Geometry check sheet. Reference: drawing and pictorial views, mm from the part's lowest x, y, z. A direction names the side the tool comes from. Coordinates: 2 decimals unless noted, no trailing zeros. Write each loop counter-clockwise with the first axis right and the second up, starting at its lowest first coordinate (ties: lowest second). Pieces come first, ordered by that corner, then holes. Notation, with made-up numbers: (16, 37) - (74, 37) arc R19 ccw to (74, 43) - close; hole circle Ø6 at (-14, -38). An arc over 180 degrees is marked (long way). Answer as CSV lines item,"result". Start each with the question number.
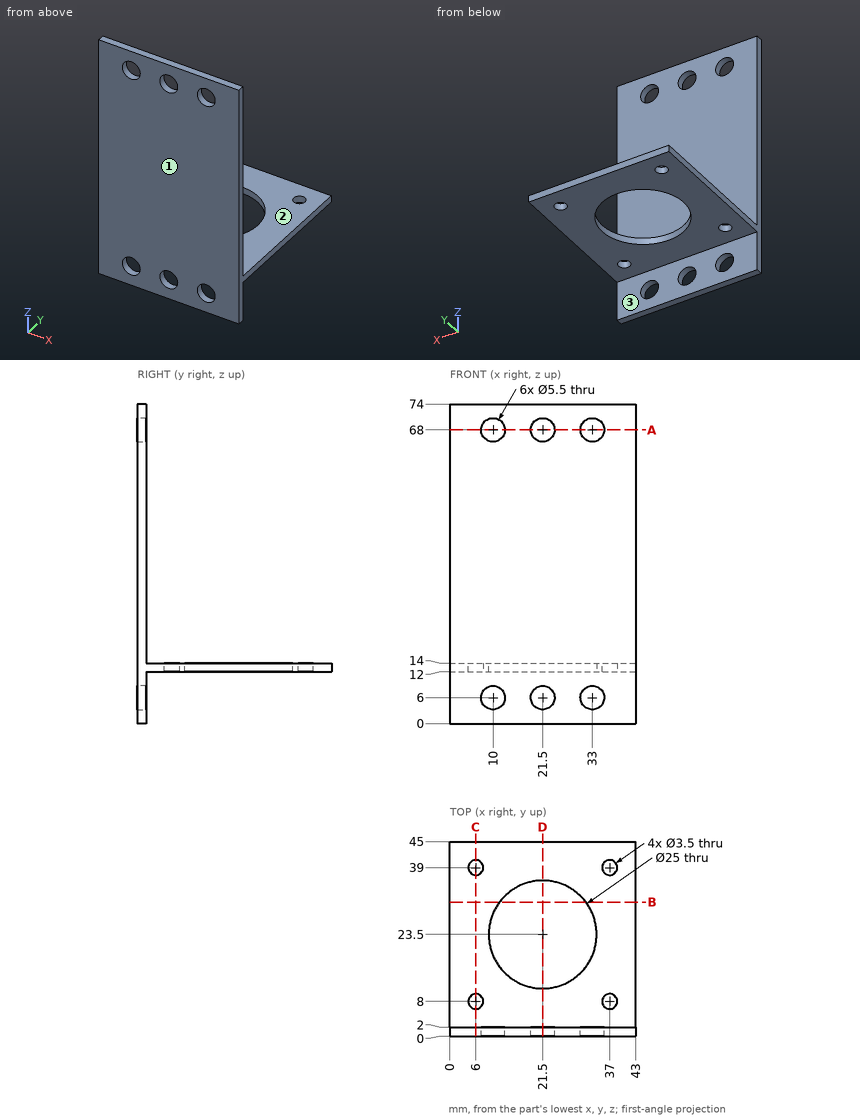
1. Cross-section at C-C (x = 6). Record the cut outline in (y, z).
2. Cross-section at A-A (z = 68). Record the cut outline in (x, y).
3. Cross-section at D-D (x = 21.5). Record the cut outline in (y, z).
4. Cross-section at B-B (y = 31). Record the cut outline in (x, z), and give its area (3 significant figures).
5. Depth check by flat-ended pin: P1, Ø10, axis at x = 13, z = 9.5, coming from the +Y side; P2, Ø13, axis at x = 19, y = 33, coming from the -Z side; P3, Ø21.5, axis at x = 14, y = 18.5, coming from the +Z side; P4, Ø7, axis at x = 33, z = 68, coming from the +Y side. Enter the tip coordinate at first touch or a pass-through.
6. Scan lines: line 1 along X through (y, z) = (0.6, 6); line 2 along Y through (x, z) = (37, 13.3); line 3 along Z through (x, y) = (8, 19.5). Record each from-to range of solid material in increasing order. Write a range as from..to.
7. Access from +Z, -Z, +X, -X, +Y, -Y to the whole of each face (thin tool, end or side, straight path). Record for the marked faces 1, 2 and 3.
Completed:
1,outline,"(0, 0) - (2, 0) - (2, 12) - (6.25, 12) - (6.25, 14) - (2, 14) - (2, 74) - (0, 74) - close; (9.75, 12) - (37.25, 12) - (37.25, 14) - (9.75, 14) - close; (40.75, 12) - (45, 12) - (45, 14) - (40.75, 14) - close"
2,outline,"(0, 0) - (7.25, 0) - (7.25, 2) - (0, 2) - close; (12.75, 0) - (18.75, 0) - (18.75, 2) - (12.75, 2) - close; (24.25, 0) - (30.25, 0) - (30.25, 2) - (24.25, 2) - close; (35.75, 0) - (43, 0) - (43, 2) - (35.75, 2) - close"
3,outline,"(0, 0) - (2, 0) - (2, 3.25) - (0, 3.25) - close; (0, 8.75) - (2, 8.75) - (2, 12) - (11, 12) - (11, 14) - (2, 14) - (2, 65.25) - (0, 65.25) - close; (0, 70.75) - (2, 70.75) - (2, 74) - (0, 74) - close; (36, 12) - (45, 12) - (45, 14) - (36, 14) - close"
4,outline,"(0, 12) - (11.5, 12) - (11.5, 14) - (0, 14) - close; (31.5, 12) - (43, 12) - (43, 14) - (31.5, 14) - close"
4,area,"46.0 mm2"
5,P1,"stops at y = 45"
5,P2,"stops at z = 12"
5,P3,"stops at z = 14"
5,P4,"stops at y = 2"
6,line 1,"x = 0..7.25, 12.75..18.75, 24.25..30.25, 35.75..43"
6,line 2,"y = 0..6.25, 9.75..37.25, 40.75..45"
6,line 3,"z = 12..14"
7,face 1,"+Z, -Z, +X, -X, -Y"
7,face 2,"+Z, +X, -X, +Y"
7,face 3,"-Z, +X, -X, +Y"
